from build123d import *

# Parameters (mm, degrees)
BOSS_EXTRUDE1_DEPTH = 25.4
FILLET1_R           = 2.54


with BuildPart() as part:
    # Sketch1 → Boss-Extrude1 (new body)
    with BuildSketch(Plane(origin=(0, 0, 0), x_dir=(1, 0, 0), z_dir=(0, 1, 0))):
        with BuildLine():
            Line((-244.848924974, -184.847069368), (-240.047965661, -181.222617027))
            ThreePointArc((-240.047965661, -181.222617027), (-245.558733938, -173.682385194), (-250.832740903, -165.974693346))
            Line((-250.832740903, -165.974693346), (-255.849395721, -169.294187212))
            ThreePointArc((-255.849395721, -169.294187212), (-250.469908617, -177.156032898), (-244.848924974, -184.847069368))
        make_face()
        with BuildLine():
            ThreePointArc((-232.905461186, -199.685956603), (-238.99238799, -192.359230601), (-244.848924974, -184.847069368))
            Line((-244.848924974, -184.847069368), (-260.051962799, -196.32450178))
            ThreePointArc((-260.051962799, -196.32450178), (-254.20265496, -203.841466748), (-248.136139057, -211.184255684))
            Line((-248.136139057, -211.184255684), (-232.905461186, -199.685956603))
        make_face()
        with BuildLine():
            ThreePointArc((-215.750093665, -209.562782535), (-228.339131483, -195.770027772), (-240.047965661, -181.222617027))
            Line((-240.047965661, -181.222617027), (-244.848924974, -184.847069368))
            ThreePointArc((-244.848924974, -184.847069368), (-238.99238799, -192.359230601), (-232.905461186, -199.685956603))
            ThreePointArc((-232.905461186, -199.685956603), (-226.594481496, -206.819670414), (-220.065095538, -213.754038186))
            Line((-220.065095538, -213.754038186), (-215.750093665, -209.562782535))
        make_face()
        with BuildLine():
            ThreePointArc((-206.580992956, -226.812099466), (-213.422935618, -220.386219322), (-220.065095538, -213.754038186))
            Line((-220.065095538, -213.754038186), (-233.729268137, -227.026347746))
            ThreePointArc((-233.729268137, -227.026347746), (-226.993847652, -233.760831798), (-220.064468162, -240.295574672))
            Line((-220.064468162, -240.295574672), (-206.580992956, -226.812099466))
        make_face()
        with BuildLine():
            ThreePointArc((-202.530385251, -222.364803398), (-209.238172175, -216.064920904), (-215.750093665, -209.562782535))
            Line((-215.750093665, -209.562782535), (-220.065095538, -213.754038186))
            ThreePointArc((-220.065095538, -213.754038186), (-213.422935618, -220.386219322), (-206.580992956, -226.812099466))
            Line((-206.580992956, -226.812099466), (-202.530385251, -222.364803398))
        make_face()
        with BuildLine():
            ThreePointArc((-188.338885995, -234.506133741), (-195.528897549, -228.545647439), (-202.530385251, -222.364803398))
            Line((-202.530385251, -222.364803398), (-206.580992956, -226.812099466))
            ThreePointArc((-206.580992956, -226.812099466), (-199.4394755, -233.116560388), (-192.105663715, -239.196256416))
            Line((-192.105663715, -239.196256416), (-188.338885995, -234.506133741))
        make_face()
    extrude(amount=BOSS_EXTRUDE1_DEPTH)

    # Fillet1
    fillet1_edges = [part.edges().sort_by_distance(p)[0] for p in [
        (-192.105663715, 12.7, 239.196256416),
        (-220.064468162, 12.7, 240.295574672),
        (-233.729268137, 12.7, 227.026347746),
        (-248.136139057, 12.7, 211.184255684),
        (-260.051962799, 12.7, 196.32450178),
        (-255.849395721, 12.7, 169.294187212),
    ]]
    fillet(fillet1_edges, radius=FILLET1_R)


solid = part.part
Input: part model. Units: mm. Frame: model coordinates. A direction names the side the tool comes from. Coordinates: 2 decimals unless noted, no trailing zeros. Order: outer loops, then holes, each group sorted by start corner. A loop starts at its lowest first (then second) coordinate and runs counter-clockwise, first axis right, second up.
1. Access query for faces 1 (the cylindrical face through (-249.8, 12.5, 178.1)), 2 (the cylindrical face through (-226.684, 12.522, 206.721)), 3 (the flat face through (-189.44, 12.52, 235.88)), 4 (the flat face through (-212.54, 12.52, 232.77)), 5 (the cylindrical face through (-227.025, 12.522, 233.731)). Directions: +Z, -Z, +X, -X, +Y, -Y. A direction counts if a zero-diameter tool reaches every point of the face in a straight line with its end or side. Return the directions, or none.
Checked values:
face 1: -X, +Y, -Y
face 2: +Y, -Y
face 3: +Z, +X, +Y, -Y
face 4: +Z, +Y, -Y
face 5: +Z, -X, +Y, -Y
2. Ray query, line 1 along Z through (x, y) = (-248, 3.5); line 2 along X through (y, z) = (19.5, 209); line 3 along X through (y, z) = (17.25, 228). Return the intervals inside material, ascending.
Checked values:
line 1: z = 170.18 to 180.6, 187.23 to 210.24
line 2: x = -249.98 to -245.24, -224.59 to -216.3
line 3: x = -232.49 to -207.77, -205.27 to -196.16
3. Contact query for flat-ended pins moving along their axis: P1, Ø8, axis at x = -198, y = 13.5, coming from the +Z side; P2, Ø1.5, axis at x = -224, y = 14.5, coming from the +Z side; P3, Ø6, axis at y = 5.5, z = 216, coming from the -X side; P4, Ø12, axis at x = -203, z = 205.5, coming from the +Y side. Output: stop coordinate, or through.
Checked values:
P1: stops at z = 237.66
P2: stops at z = 237.34
P3: stops at x = -225.47
P4: passes through
4. Cut plane A-A, the plane x = -221. Return loops of the section in (y, z).
Checked values:
outline: (0, 204.02) - (25.4, 204.02) - (25.4, 212.79) - (0, 212.79) - close; (0, 214.66) - (25.4, 214.66) - (25.4, 239.16) - (0, 239.16) - close
5. Cut plane D-D, the plane z = 191. Return loops of the section in (x, y).
Checked values:
outline: (-253, 0) - (-232.34, 0) - (-232.34, 25.4) - (-253, 25.4) - close
6. Draft query along X for faces 6 (the cylindrical face through (-254.806, 12.878, 169.481)), 7 (the cylindrical face through (-220.116, 12.878, 239.314)), 8 (the cylindrical face through (-200.498, 12.522, 232.207)). Return one class per face: +X half, -X half, draft (parallel to the pull), parting line (faces both ways), or undercut.
Checked values:
face 6: -X half
face 7: parting line
face 8: undercut
7. Cut plane C-C, the plane z = 230. Return loops of the section in (x, y), plus the area to 3 significant figures.
Checked values:
outline: (-230.8, 0) - (-209.77, 0) - (-209.77, 25.4) - (-230.8, 25.4) - close; (-203.03, 0) - (-193.82, 0) - (-193.82, 25.4) - (-203.03, 25.4) - close
area: 768 mm2
8. Cut plane B-B, the plane y = 9.5. Return loops of the section in (x, z), plus the area to 3 significant figures.
Checked values:
outline: (-258.5, 198.36) arc R2.54 ccw to (-258.02, 194.79) - (-244.85, 184.85) arc R306.79 ccw to (-254.43, 171.42) arc R2.54 ccw to (-253.72, 167.89) - (-250.83, 165.97) arc R300.77 cw to (-188.34, 234.51) - (-190.51, 237.21) arc R2.54 ccw to (-194.1, 237.58) arc R306.79 ccw to (-206.58, 226.81) - (-218.34, 238.57) arc R2.54 ccw to (-221.86, 238.63) arc R325.84 ccw to (-231.94, 228.86) arc R2.54 ccw to (-231.9, 225.25) - (-220.07, 213.75) arc R306.79 ccw to (-232.91, 199.69) - (-246.22, 209.74) arc R2.54 ccw to (-249.69, 209.34) arc R325.84 ccw to start
area: 1,280 mm2
